The listing builds one solid part. Answer for the finished solid, in the listing's coordinates (mm). Face numbers are marked on the shaded views. A direction names the side the tool comes from. Round coordinates to 2 decimals unless told otherwise and drop trailing zeros. Write each loop counter-clockwise with the first axis right and the second up, starting at its lowest first coordinate (ties: lowest second). Pieces come first, ordered by that corner, then holes.
(1) A cutting plane is placed at A-A, the plane y = -40.5. Give the vertices of the cut face in (x, z), and give its area (3 significant figures).
(2) Find the intervals of material crossed by probe 1 along Z at (x, y) = (98, -83); probe 2 along Z at (x, y) = (93, -321.5); probe 3 along Y at (x, z) = (139.5, 185.5), in increasing order.
(3) Each of these flat-tipped pins is pushed along its axis until it touches: pin 1 Ø5 at (x, y) = (153.5, -82) entering from +Z; pin 2 Ø4 at (x, z) = (87.5, 72.5) entering from +Y; pin 3 Ø1.5 at (x, y) = (104, -242) entering from -Z. Where does it stop, or does it pass through?
(4) For the marked faces 5, 6 and 7, determine the directions among +Z, -Z, +X, -X, +Y, -Y from which every point of the face is accessible in a straight line to the end or side of a thin tool.
(5) The mould has two halves that part along Z. Classify the marked faces 1, 2, 3 and 4: +Z half, -Z half, draft (parallel to the pull), parting line (faces both ways), or undercut.
(6) A cutting plane is placed at C-C, the plane z = -71.5. Give the vertices of the cut face in (x, y).
(7) A cutting plane is placed at B-B, the plane x = -47. Give the vertices of the cut face in (y, z).
(8) A cutting plane is placed at D-D, the plane y = 205. Give the vertices of the cut face in (x, z).
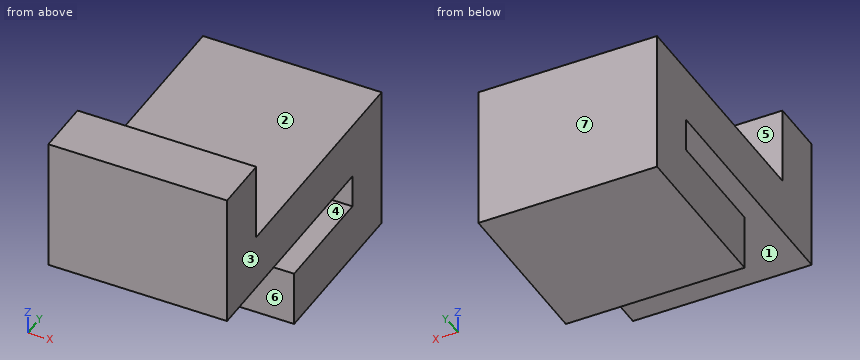
from build123d import *

# Parameters (mm, degrees)
BOSS_EXTRUDE1_DEPTH = 203.2


with BuildPart() as part:
    # Sketch1 → Boss-Extrude1 (new body, symmetric)
    with BuildSketch(Plane(origin=(0, 0, 0), x_dir=(0, 0, -1), z_dir=(1, 0, 0))):
        Polygon((-241.3, -273.05), (-63.5, -273.05), (-63.5, 273.05), (63.5, 273.05), (266.7, 273.05), (266.7, 146.05), (266.7, -107.95), (139.7, -107.95), (139.7, 146.05), (63.5, 146.05), (63.5, -273.05), (63.5, -400.05), (-241.3, -400.05), align=None)
    extrude(amount=BOSS_EXTRUDE1_DEPTH, both=True)


solid = part.part
Solutions:
1. outline: (-203.2, -266.7) - (203.2, -266.7) - (203.2, -139.7) - (-203.2, -139.7) - close; (-203.2, -63.5) - (203.2, -63.5) - (203.2, 63.5) - (-203.2, 63.5) - close
1. area: 103,000 mm2
2. probe 1: z = -266.7 to -139.7, -63.5 to 63.5
2. probe 2: z = -63.5 to 241.3
2. probe 3: y = -400.05 to -273.05
3. pin 1: stops at z = 63.5
3. pin 2: stops at y = -273.05
3. pin 3: stops at z = -63.5
4. face 5: +Z, +X, -X, +Y
4. face 6: -Z, +X, -X, -Y
4. face 7: +Z, -Z, +X, -X, +Y
5. face 1: undercut
5. face 2: +Z half
5. face 3: draft
5. face 4: undercut
6. outline: (-203.2, 146.05) - (203.2, 146.05) - (203.2, 273.05) - (-203.2, 273.05) - close
7. outline: (-400.05, -63.5) - (146.05, -63.5) - (146.05, -139.7) - (-107.95, -139.7) - (-107.95, -266.7) - (273.05, -266.7) - (273.05, 63.5) - (-273.05, 63.5) - (-273.05, 241.3) - (-400.05, 241.3) - close
8. outline: (-203.2, -266.7) - (203.2, -266.7) - (203.2, 63.5) - (-203.2, 63.5) - close
